Solid Edge part; units mm, degrees
extrude "Protrusion1" [suppressed]
extrude "Extrusionsausschnitt_1" [suppressed]
extrude "Extrusionsausprägung_2" [suppressed]
extrude "Protrusion2" [suppressed]
extrude "Extrusionsausprägung_4" [suppressed]
extrude "Extrusionsausschnitt_2" [suppressed]
extrude "Extrusionsausschnitt_3" [suppressed]
extrude "Extrusionsausschnitt_4" [suppressed]
sketch "Sketch1" plane through (0, 1.5, 0) normal (0, 0, 1) x (0, 1, 0)
  line L0 (-21.5005, 26.9994) -> (-21.5005, -26.9994)
  line L1 (-21.5005, -26.9994) -> (21.5005, -26.9994)
  line L2 (21.5005, -26.9994) -> (21.5005, 26.9994)
  line L3 (21.5005, 26.9994) -> (-21.5005, 26.9994)
extrude "Protrusion3" add sketch "Sketch1" along normal blind 20
sketch "Sketch2" plane through (0, 1.5, 0) normal (0, 0, -1) x (0, 1, 0)
  line L0 (-20.5005, -25.9994) -> (17.5005, -25.9994)
  line L1 (17.5005, -25.9994) -> (17.5005, 25.9994)
  line L2 (17.5005, 25.9994) -> (-20.5005, 25.9994)
  line L3 (-20.5005, 25.9994) -> (-20.5005, -25.9994)
extrude "Extrusionsausschnitt_5" cut sketch "Sketch2" against normal blind 19
sketch "Sketch3" plane through (0, 1.5, 0) normal (0, 0, -1) x (-1, 0, 0)
  line L0 (-19.993, 17.5005) -> (20.007, 17.5005)
  line L1 (20.007, 17.5005) -> (20.007, 20.0005)
  line L2 (20.007, 20.0005) -> (-19.993, 20.0005)
  line L3 (-19.993, 20.0005) -> (-19.993, 17.5005)
  dimension "D1" = 20.007
  dimension "D2" = 20.007
extrude "Extrusionsausschnitt_6" cut sketch "Sketch3" against normal blind 17.5
sketch "Sketch4" plane through (0, 1.5, 0) normal (0, 0, -1) x (-1, 0, 0)
  line L0 (-16.7505, 20.0005) -> (16.7495, 20.0005)
  line L1 (16.7495, 20.0005) -> (16.7495, 21.5005)
  line L2 (16.7495, 21.5005) -> (-16.7505, 21.5005)
  line L3 (-16.7505, 21.5005) -> (-16.7505, 20.0005)
  dimension "D1" = 16.7495
extrude "Extrusionsausschnitt_7" cut sketch "Sketch4" against normal blind 14
sketch "Sketch5" plane through (0, 1.5, 0) normal (0, 0, -1) x (0, -1, 0)
  line L0 (-1.2155, 26.9994) -> (14.7845, 26.9994)
  line L1 (14.7845, 26.9994) -> (14.7845, 25.9994)
  line L2 (14.7845, 25.9994) -> (-1.2155, 25.9994)
  line L3 (-1.2155, 25.9994) -> (-1.2155, 26.9994)
extrude "Extrusionsausschnitt_8" cut sketch "Sketch5" against normal blind 13
sketch "Sketch6" plane through (0, 1.5, 0) normal (0, 0, -1) x (0, -1, 0)
  line L0 (18.7753, -18.5802) -> (21.5005, -18.5802)
  line L1 (21.5005, -18.5802) -> (21.5005, -9.9402)
  line L2 (21.5005, -9.9402) -> (18.7753, -9.9402)
  line L3 (18.7753, -9.9402) -> (18.7753, -18.5802)
extrude "Extrusionsausschnitt_9" cut sketch "Sketch6" against normal blind 4
sketch "Sketch7" plane through (0, 0, 19) normal (0, 0, -1) x (0, -1, 0)
  line L0 (-19.0496, 20.9493) -> (-13.9496, 20.9493)
  line L1 (-13.9496, 20.9493) -> (-13.9496, 26.0493)
  line L2 (-13.9496, 26.0493) -> (-19.0496, 26.0493)
  line L3 (-19.0496, 26.0493) -> (-19.0496, 20.9493)
  line L4 (13.9506, 20.9493) -> (19.0506, 20.9493)
  line L5 (19.0506, 20.9493) -> (19.0506, 26.0493)
  line L6 (19.0506, 26.0493) -> (13.9506, 26.0493)
  line L7 (13.9506, 26.0493) -> (13.9506, 20.9493)
  line L8 (13.9506, -26.0506) -> (19.0506, -26.0506)
  line L9 (19.0506, -26.0506) -> (19.0506, -20.9506)
  line L10 (19.0506, -20.9506) -> (13.9506, -20.9506)
  line L11 (13.9506, -20.9506) -> (13.9506, -26.0506)
  line L12 (-19.0496, -26.0506) -> (-13.9496, -26.0506)
  line L13 (-13.9496, -26.0506) -> (-13.9496, -20.9506)
  line L14 (-13.9496, -20.9506) -> (-19.0496, -20.9506)
  line L15 (-19.0496, -20.9506) -> (-19.0496, -26.0506)
extrude "Extrusionsausprägung_6" add sketch "Sketch7" along normal blind 19
sketch "Sketch8" plane through (-23.4744, -16.4755, 0) normal (0, 0, -1) x (0, -1, 0)
  circle A0 centre (0.0251, 0.0249) radius 1.1
  circle A1 centre (0.0251, -46.975) radius 1.1
  circle A2 centre (-32.9751, -46.975) radius 1.1
  circle A3 centre (-32.9751, 0.0249) radius 1.1
extrude "Cutout1" cut sketch "Sketch8" against normal blind 10
sketch "Sketch9" plane through (-21.9995, 12.858, 0) normal (0, 0, -1) x (0, -1, 0)
  line L0 (-9.9425, 10.0509) -> (-9.9425, -54.0498)
extrude "Extrusionsausschnitt_11" cut sketch "Sketch9" along normal mid plane 152.9747 material side at (-0.0001, 22.8505, 0)
sketch "Sketch10" plane through (0, 22.8005, 10) normal (0, 1, 0) x (-1, 0, 0)
  line L0 (-26.9994, 10) -> (-26.9994, -10)
  line L1 (-26.9994, -10) -> (-16.7505, -10)
  line L2 (-16.7505, -10) -> (-16.7505, 4)
  line L3 (-16.7505, 4) -> (16.7495, 4)
  line L4 (16.7495, 4) -> (16.7495, -10)
  line L5 (16.7495, -10) -> (26.9994, -10)
  line L6 (26.9994, -10) -> (26.9994, 10)
  line L7 (26.9994, 10) -> (-26.9994, 10)
extrude "Protrusion4" add sketch "Sketch10" along normal blind 0.5
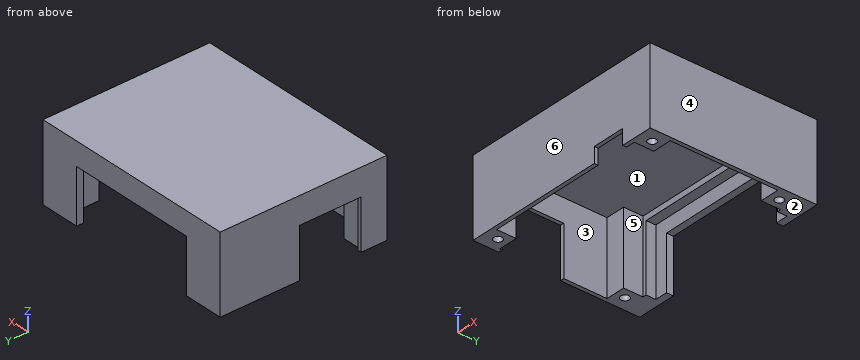
Geometry: final body of the model. Coordinates: model frame, mm. Face numbers are marked on the shaded views. A direction names the side the tool comes from. Round coordinates to 2 decimals unless told otherwise and drop trailing zeros. Loops run counter-clockwise (first coordinate to the right, second up) from the corner with the lowest first, then second, coordinate; pieces in that order, holes last. Notation, with made-up numbers: (54.5, 6) -> (85.5, 6) arc R20 cw to (85.5, 45) -> close; hole circle Ø6 at (71.25, 12). An arc over 180 degrees is marked (long way). Use one line per item in the form item = value.
Item 1: Material intervals for probe 1 along X at (y, z) = (6, 2.5); probe 2 along Y at (x, z) = (-21.5, 17); probe 3 along Y at (x, z) = (14, 15.5), sorted ascending.
Evaluation:
probe_1 = -27 to -26, 26 to 27
probe_2 = -20 to -13.95, 13.95 to 23.3
probe_3 = -20 to -19, 21.5 to 23.3
Item 2: Cut plane B-B on y = -5. Output: boundary loops of the cut face in (x, z).
Evaluation:
outline = (-27, 13) -> (-26, 13) -> (-26, 19) -> (26, 19) -> (26, 0) -> (27, 0) -> (27, 20) -> (-27, 20) -> close
Item 3: Cut plane C-C on z = 15.75. Output: boundary loops of the cut face in (x, y), then the cut area to 3 significant figures.
Evaluation:
outline = (-27, -20) -> (27, -20) -> (27, 23.3) -> (-27, 23.3) -> close; hole (-26, -13.95) -> (-20.95, -13.95) -> (-20.95, -19) -> (20.95, -19) -> (20.95, -13.95) -> (26, -13.95) -> (26, 13.95) -> (20.95, 13.95) -> (20.95, 19) -> (19.99, 19) -> (19.99, 21.5) -> (-20.01, 21.5) -> (-20.01, 19) -> (-20.95, 19) -> (-20.95, 13.95) -> (-26, 13.95) -> close
area = 364 mm2
Item 4: Access query for the marked faces 5 and 6. Directions: +Z, -Z, +X, -X, +Y, -Y. A direction counts if a zero-diameter tool reaches every point of the face in a straight line with its end or side. Return the directions, or none.
Evaluation:
face_5 = -Z
face_6 = +Z, -Z, +X, -X, -Y
Item 5: Contact query for flat-ended pins moving along their axis: pin 1 Ø1.1 at (x, y) = (-26.5, -6) entering from -Z; pin 2 Ø5.5 at (x, z) = (0, 11) entering from +Y; pin 3 Ø1.8 at (x, y) = (23.5, -16.5) entering from -Z; pin 4 Ø12 at (y, z) = (0, 6) entering from -X. Output: stop coordinate, or through.
Evaluation:
pin_1 = 13
pin_2 = -19
pin_3 = 10
pin_4 = -27
Item 6: Cut plane A-A on z = 11.5. Output: boundary loops of the cut face in (x, y), then the cut area to 3 significant figures.
Evaluation:
outline = (-27, -20) -> (27, -20) -> (27, 23.3) -> (16.75, 23.3) -> (16.75, 21.5) -> (19.99, 21.5) -> (19.99, 19) -> (20.95, 19) -> (20.95, 13.95) -> (26, 13.95) -> (26, -13.95) -> (20.95, -13.95) -> (20.95, -19) -> (-20.95, -19) -> (-20.95, -13.95) -> (-26, -13.95) -> (-26, -13.28) -> (-27, -13.28) -> close; (-27, 2.72) -> (-26, 2.72) -> (-26, 13.95) -> (-20.95, 13.95) -> (-20.95, 19) -> (-20.01, 19) -> (-20.01, 21.5) -> (-16.75, 21.5) -> (-16.75, 23.3) -> (-27, 23.3) -> close
area = 288 mm2
Item 7: Cut plane D-D on x = -6. Output: boundary loops of the cut face in (y, z), then the cut area to 3 significant figures.
Evaluation:
outline = (-20, 0) -> (-19, 0) -> (-19, 19) -> (19, 19) -> (19, 17.5) -> (21.5, 17.5) -> (21.5, 14) -> (23.3, 14) -> (23.3, 20) -> (-20, 20) -> close
area = 75.1 mm2
Item 8: Draft query along X for the marked faces 1, 2, 3 and 4. Return one class per face: released by +X, released by -X, zero draft, split by the parting line, or undercut.
Evaluation:
face_1 = undercut
face_2 = zero draft
face_3 = undercut
face_4 = released by +X
